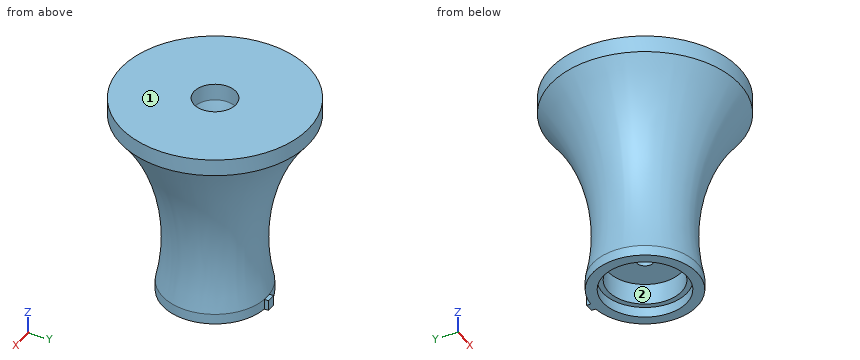
```python
from build123d import *

# Parameters (mm, degrees)
F3_DEPTH  = 4.9
F4_R      = 20
F4_R_2    = 4
F5_DEPTH  = 4.9
F6_DEPTH  = 8
F7_R      = 17.5
F8_DEPTH  = 10
F10_DEPTH = 5


with BuildPart() as f2:
    # F0 (on Front) → F2 (revolve)
    with BuildSketch(Plane.XZ):
        with BuildLine():
            Line((4, 0), (25, 0))
            ThreePointArc((25, 0), (25.0633115181, 44.8380443487), (45, 85))
            Line((45, 85), (10, 85))
            ThreePointArc((10, 85), (5.5209994492, 72.8549601322), (4, 60))
            Line((4, 60), (4, 0))
        make_face()
    revolve(axis=Axis((0, 0, 25.1682717353), (0, 0, 1)))

    # F3 (add): a face of the model
    f3_faces = [f2.faces().sort_by_distance(p)[0] for p in [
        (-4.7071067812, 0, 0),
    ]]
    extrude(f3_faces, amount=F3_DEPTH)

    # F4 (on face) → F5 (cut)
    with BuildSketch(Plane(origin=(0, 0, -4.9), x_dir=(1, 0, 0), z_dir=(0, 0, -1))):
        Circle(F4_R)
        Circle(F4_R_2, mode=Mode.SUBTRACT)
    extrude(amount=-F5_DEPTH, mode=Mode.SUBTRACT)

    # F6 (add): a face of the model
    f6_faces = [f2.faces().sort_by_distance(p)[0] for p in [
        (-43.7272077939, 0, 85),
    ]]
    extrude(f6_faces, amount=F6_DEPTH)

    # F7 (on Top) → F8 (cut)
    with BuildSketch(Plane.XY):
        Circle(F7_R)
    extrude(amount=F8_DEPTH, mode=Mode.SUBTRACT)

    # F9 (on face) → F10 (join)
    with BuildSketch(Plane(origin=(0, 0, -4.9), x_dir=(1, 0, 0), z_dir=(0, 0, -1))):
        with BuildLine():
            ThreePointArc((2.125, -24.9095237811), (0, -25), (-2.125, -24.9095237811))
            Line((-2.125, -24.9095237811), (-2.125, -26.9095237811))
            Line((-2.125, -26.9095237811), (2.125, -26.9095237811))
            Line((2.125, -26.9095237811), (2.125, -24.9095237811))
        make_face()
    extrude(amount=-F10_DEPTH)


solid = f2.part
```
Design review of the part built by this model. Coordinates are the model's own, in mm. Face numbers are marked on the shaded views. Coordinates: 2 decimals unless noted, no trailing zeros. Loops run counter-clockwise (first coordinate to the right, second up) from the corner with the lowest first, then second, coordinate; pieces in that order, holes last.
Q1. We need section B-B on x = 0. State the section outline as (y, z) points, and give its area (3 significant figures).
Reported:
outline: (-45, 85) arc R98.47 cw to (-25, 0) - (-25, -4.9) - (-20, -4.9) - (-20, 0) - (-17.5, 0) - (-17.5, 10) - (-4, 10) - (-4, 60) arc R55.08 ccw to (-10, 85) - (-10, 93) - (-45, 93) - close; (4, 10) - (17.5, 10) - (17.5, 0) - (20, 0) - (20, -4.9) - (26.91, -4.9) - (26.91, 0.1) - (25, 0.1) - (25, 0) arc R98.47 cw to (45, 85) - (45, 93) - (10, 93) - (10, 85) arc R55.08 ccw to (4, 60) - close
area: 4,320 mm2
Q2. For pin 1 (5 mm diameter, centred on x = -3, y = 32.5, fed in from -Z); pin 2 (1 mm diameter, centred on y = 26.5, z = -2.5, fed in from -X) (3 decimals); pin 3 (2 mm diameter, centred on x = 0, z = -1.5, fed in from +Y), all flat-tipped, find the tip position at first contact; note any pin that passes through.
Reported:
pin 1: stops at z = 60.44
pin 2: stops at x = -2.125
pin 3: stops at y = 26.91
Q3. We need section A-A on y = 0. State the section outline as (x, z) points, and give its area (3 significant figures).
Reported:
outline: (-45, 85) arc R98.47 cw to (-25, 0) - (-25, -4.9) - (-20, -4.9) - (-20, 0) - (-17.5, 0) - (-17.5, 10) - (-4, 10) - (-4, 60) arc R55.08 ccw to (-10, 85) - (-10, 93) - (-45, 93) - close; (4, 10) - (17.5, 10) - (17.5, 0) - (20, 0) - (20, -4.9) - (25, -4.9) - (25, 0) arc R98.47 cw to (45, 85) - (45, 93) - (10, 93) - (10, 85) arc R55.08 ccw to (4, 60) - close
area: 4,310 mm2
Q4. We need section D-D on z = 11.5. State the section outline as (x, y) points.
Reported:
outline: circle Ø46.08 at (0, 0); hole circle Ø8 at (0, 0)
Q5. To check wall thickness, follow line 1 (Y direction, x = 0, z = -2); line 2 (Y direction, x = 0, z = 89); line 3 (X direction, y = 0, z = -1.55). State the ranges of each line that lie inside material, in increasing order.
Reported:
line 1: y = -25 to -20, 20 to 26.91
line 2: y = -45 to -10, 10 to 45
line 3: x = -25 to -20, 20 to 25
Q6. The part is to be moulded in two halves that separate along X. For the marked faces 1 and 2, say which applies: +X half, -X half, draft (parallel to the pull), parting line (faces both ways), or undercut.
Reported:
face 1: draft
face 2: undercut
Q7. We need section C-C on z = 73. State the section outline as (x, y) points.
Reported:
outline: circle Ø73.02 at (0, 0); hole circle Ø11.11 at (0, 0)
